Can you work these out from the model? Positions are in its coordinate system, mm. A direction names the side the tool comes from. Give positions to 0.01 mm unless a question says otherwise; leave off trailing zeros. Loops run counter-clockwise (first coordinate to the right, second up) from the corner with the lowest first, then second, coordinate; pieces in that order, holes last. Notation, with made-up numbers: (21, 1) -> (29, 1) arc R16 cw to (29, 16) -> close; hole circle Ø2 at (63, 38.25). An arc over 180 degrees is marked (long way). Return JSON: item names as keys, results as strings. Group by question number.
Q1. Thinking about a two-plate mould opening in X: for faces 6 (the flat face through (0, 0, -2)), 7 (the flat face through (0.5, 2, -4)), 8 (the flat face through (-4.1, 2.19, 1.79)), which applies, pulls with the +X half, pulls with the -X half, needs draft (parallel to the pull), parting line crosses it, or undercut?
Q2. Suppose I cut it at A-A, the plane y = 1. Please give me the cut outline in (x, z), and give its area (3 significant figures).
Q3. Which directions (+Z, -Z, +X, -X, +Y, -Y) give clear straight access to the entire face, cutting with the end or side of a thin tool? Please do faces 1 (the flat face through (4.1, 2.19, 1.79)), 2 (the flat face through (5, 9.5, 5)), 3 (the flat face through (-4.1, 2.19, -1.79)), 4 (the flat face through (-0.5, 2, 4)), 5 (the flat face through (-3.602, 2.193, -2.657)).
Q4. Will these pins go through, and if not, where does the flat tip stop? pin 1 (8 mm diameter, centred on y = 10.5, z = 10.5, fed in from +X); pin 2 (8 mm diameter, centred on x = 6, y = 8, fed in from +Z); pin 3 (2 mm diameter, centred on x = -18.19, z = 10.5, fed in from -Y).
Q5. I need wall thicknesses on line 1 along X through (y, z) = (13.15, 10.5); line 2 along X through (y, z) = (10, 5); line 3 along Y through (x, z) = (0.5, 12). Which ranges of each line are inside material? Lowest first, please. Write a range as [from, to].
Q6. Suppose I cut it at B-B, the plane y = 11.5. Count the separate pieces of the cut face and the enclosed holes in it, and give its area (3 significant figures).
```python
from build123d import *

# Parameters (mm, degrees)
BOSS_EXTRUDE2_REACH = 44.382
SKETCH3_W           = 1
SKETCH3_H           = 6.5
CIRPATTERN1_COUNT   = 6
SKETCH5_R           = 0.75
CUT_EXTRUDE1_DEPTH  = 39.213217609
CIRPATTERN2_COUNT   = 6
SKETCH6_R           = 0.75
CUT_EXTRUDE2_DEPTH  = 39.213217609
CHAMFER1_SIZE       = 0.5


with BuildPart() as part:
    # Sketch1 → Revolve1 (revolve)
    with BuildSketch(Plane.XY, mode=Mode.PRIVATE) as revolve1_sk:
        Polygon((1.6, 0), (2, 0), (6.551348998, 6.5), (6.551348998, 9.5), (25, 9.5), (25, 14.5), (3, 14.5), (3, 5.2), (1.6, 3.8), align=None)
    revolve(revolve1_sk.sketch.rotate(Axis((0, 0, 0), (0, 1, 0)), 90), axis=Axis((0, 0, 0), (0, 1, 0)))

    # Sketch3 → Boss-Extrude2 (add, up to next)
    with BuildSketch(Plane.XY.offset(6), mode=Mode.PRIVATE) as boss_extrude2_sk1:
        with Locations((0, 3.25)):
            Rectangle(SKETCH3_W, SKETCH3_H)
    boss_extrude2_tool1 = extrude(boss_extrude2_sk1.sketch, amount=-BOSS_EXTRUDE2_REACH, mode=Mode.PRIVATE) - part.part
    boss_extrude2 = boss_extrude2_tool1.solids().sort_by_distance((0, 3.25, 6))[0]
    add(boss_extrude2)

    # CirPattern1: Boss-Extrude2 ×6 about axis
    cirpattern1_axis = Axis((0, 0, 0), (0, 1, 0))
    for i in range(1, CIRPATTERN1_COUNT):
        add(boss_extrude2.rotate(cirpattern1_axis, i * 360 / CIRPATTERN1_COUNT))

    # Sketch5 → Cut-Extrude1 (cut, through all)
    with BuildSketch(Plane(origin=(0, 14.5, 0), x_dir=(1, 0, 0), z_dir=(0, 1, 0))):
        with Locations(Location((0, 21, 0), (0, 0, 270))):
            Circle(SKETCH5_R)
    cut_extrude1 = extrude(amount=-CUT_EXTRUDE1_DEPTH, mode=Mode.SUBTRACT)

    # CirPattern2: Cut-Extrude1 ×6 about axis
    cirpattern2_axis = Axis((0, 0, 0), (0, 1, 0))
    for i in range(1, CIRPATTERN2_COUNT):
        add(cut_extrude1.rotate(cirpattern2_axis, i * 360 / CIRPATTERN2_COUNT), mode=Mode.SUBTRACT)

    # Sketch6 → Cut-Extrude2 (cut, through all)
    with BuildSketch(Plane(origin=(0, 14.5, 0), x_dir=(1, 0, 0), z_dir=(0, 1, 0))):
        with Locations(Location((-10, 15, 0), (0, 0, 270))):
            Circle(SKETCH6_R)
        with Locations(Location((10, 15, 0), (0, 0, 270))):
            Circle(SKETCH6_R)
        with Locations(Location((-10, -15, 0), (0, 0, 270))):
            Circle(SKETCH6_R)
        with Locations(Location((10, -15, 0), (0, 0, 270))):
            Circle(SKETCH6_R)
    extrude(amount=-CUT_EXTRUDE2_DEPTH, mode=Mode.SUBTRACT)

    # Chamfer1
    chamfer1_edges = [part.edges().sort_by_distance(p)[0] for p in [
        (0, 14.5, 3),
        (0, 14.5, 25),
        (0, 9.5, 25),
    ]]
    chamfer(chamfer1_edges, length=CHAMFER1_SIZE)


solid = part.part
```
Ans:
{
 "1": {"face 6": "needs draft", "face 7": "undercut", "face 8": "pulls with the -X half"},
 "2": {"outline": "(-5.45, -2.57) -> (-4.95, -3.43) -> (-2.05, -1.76) arc R2.7 ccw to (-0.5, -2.65) -> (-0.5, -6) -> (0.5, -6) -> (0.5, -2.65) arc R2.7 ccw to (2.05, -1.76) -> (4.95, -3.43) -> (5.45, -2.57) -> (2.55, -0.89) arc R2.7 ccw to (2.55, 0.89) -> (5.45, 2.57) -> (4.95, 3.43) -> (2.05, 1.76) arc R2.7 ccw to (0.5, 2.65) -> (0.5, 6) -> (-0.5, 6) -> (-0.5, 2.65) arc R2.7 ccw to (-2.05, 1.76) -> (-4.95, 3.43) -> (-5.45, 2.57) -> (-2.55, 0.89) arc R2.7 ccw to (-2.55, -0.89) -> close; hole circle Ø3.2 at (0, 0)", "area": "34.8 mm^2"},
 "3": {"face 1": "+X, -Y", "face 2": "-Y", "face 3": "-X, -Y", "face 4": "+Z, -Y", "face 5": "-Z, -Y"},
 "4": {"pin 1": "stops at x = 24.14", "pin 2": "stops at z = 24.87", "pin 3": "stops at y = 9.5"},
 "5": {"line 1": "x = [-22.69, -18.94], [-17.44, 17.44], [18.94, 22.69]", "line 2": "x = [-24.49, 24.49]", "line 3": "y = [9.5, 14.5]"},
 "6": {"separate pieces": "1", "enclosed holes": "11", "area": "1,920 mm^2"}
}
